from build123d import *

# Parameters (mm, degrees)
SKETCH2_R           = 27.5
BOSS_EXTRUDE1_DEPTH = 3.175
SKETCH3_R           = 1.5
SKETCH3_R_2         = 1.25
SKETCH3_W           = 3.81
SKETCH3_H           = 1.5
CUT_EXTRUDE1_DEPTH  = 3.175
SKETCH4_W           = 3.5
SKETCH4_H           = 4.54
CUT_EXTRUDE2_DEPTH  = 10
SKETCH5_W           = 19
SKETCH5_H           = 6
SKETCH5_W_2         = 12.7
SKETCH5_H_2         = 5.1
CUT_EXTRUDE3_DEPTH  = 10


with BuildPart() as part:
    # Sketch2 → Boss-Extrude1 (new body)
    with BuildSketch(Plane(origin=(0, 0, 0), x_dir=(1, 0, 0), z_dir=(0, 1, 0))):
        with Locations(Location((0, 0, 0), (0, 0, 270))):
            Circle(SKETCH2_R)
    extrude(amount=BOSS_EXTRUDE1_DEPTH)

    # Sketch3 → Cut-Extrude1 (cut)
    with BuildSketch(Plane(origin=(0, 3.175, 0), x_dir=(1, 0, 0), z_dir=(0, 1, 0))):
        with Locations((-4.7, 20.68)):
            Circle(SKETCH3_R)
        with Locations(Location((0, 15, 0), (0, 0, 270))):
            Circle(SKETCH3_R_2)
        with Locations(Location((-12.990381057, -7.5, 0), (0, 0, 270))):
            Circle(SKETCH3_R_2)
        with Locations(Location((12.990381057, -7.5, 0), (0, 0, 270))):
            Circle(SKETCH3_R_2)
        with BuildLine():
            Line((-1.90505, 20.68), (-1.90505, 22.18))
            Line((-1.90505, 22.18), (-4.7, 22.18))
            ThreePointArc((-4.7, 22.18), (-3.639339828, 21.740660172), (-3.2, 20.68))
            ThreePointArc((-3.2, 20.68), (-3.639339828, 19.619339828), (-4.7, 19.18))
            Line((-4.7, 19.18), (-1.174368952, 19.18))
            ThreePointArc((-1.174368952, 19.18), (-1.71266534, 19.845749619), (-1.90505, 20.68))
        make_face()
        with BuildLine():
            Line((1.90495, 20.68), (-1.90505, 20.68))
            ThreePointArc((-1.90505, 20.68), (-1.71266534, 19.845749619), (-1.174368952, 19.18))
            Line((-1.174368952, 19.18), (1.174268952, 19.18))
            ThreePointArc((1.174268952, 19.18), (1.71256534, 19.845749619), (1.90495, 20.68))
        make_face()
        with Locations((-5e-05, 21.43)):
            Rectangle(SKETCH3_W, SKETCH3_H)
        with BuildLine():
            Line((4.7, 22.18), (1.90495, 22.18))
            Line((1.90495, 22.18), (1.90495, 20.68))
            ThreePointArc((1.90495, 20.68), (1.71256534, 19.845749619), (1.174268952, 19.18))
            Line((1.174268952, 19.18), (4.7, 19.18))
            ThreePointArc((4.7, 19.18), (3.2, 20.68), (4.7, 22.18))
        make_face()
        with Locations((4.7, 20.68)):
            Circle(SKETCH3_R)
        with Locations((-15.55940535, -14.410319398)):
            Circle(SKETCH3_R)
        with BuildLine():
            ThreePointArc((-15.750561777, -11.079226754), (-16.027379451, -11.399040856), (-16.367944576, -11.649888379))
            Line((-16.367944576, -11.649888379), (-18.255879956, -12.739888379))
            Line((-18.255879956, -12.739888379), (-16.858443456, -15.160319398))
            ThreePointArc((-16.858443456, -15.160319398), (-16.30940535, -13.111281292), (-14.260367245, -13.660319398))
            Line((-14.260367245, -13.660319398), (-15.750561777, -11.079226754))
        make_face()
        Polygon((-18.255879956, -12.739888379), (-16.367944576, -11.649888379), (-18.272944576, -8.350331591), (-20.160879956, -9.440331591), align=None)
        with BuildLine():
            Line((-18.272944576, -8.350331591), (-16.367944576, -11.649888379))
            ThreePointArc((-16.367944576, -11.649888379), (-16.027379451, -11.399040856), (-15.750561777, -11.079226754))
            Line((-15.750561777, -11.079226754), (-17.470045712, -8.100993217))
            ThreePointArc((-17.470045712, -8.100993217), (-17.885421686, -8.180817303), (-18.272944576, -8.350331591))
        make_face()
        with BuildLine():
            Line((-20.160879956, -9.440331591), (-18.272944576, -8.350331591))
            ThreePointArc((-18.272944576, -8.350331591), (-17.885421686, -8.180817303), (-17.470045712, -8.100993217))
            Line((-17.470045712, -8.100993217), (-18.960367245, -5.519680602))
            ThreePointArc((-18.960367245, -5.519680602), (-18.810516611, -5.881452035), (-18.75940535, -6.269680602))
            ThreePointArc((-18.75940535, -6.269680602), (-19.871176783, -7.718569342), (-21.558443456, -7.019680602))
            Line((-21.558443456, -7.019680602), (-20.160879956, -9.440331591))
        make_face()
        with Locations((-20.25940535, -6.269680602)):
            Circle(SKETCH3_R)
        with BuildLine():
            ThreePointArc((17.470087928, -8.100920096), (17.888564549, -8.181681202), (18.278613112, -8.353457675))
            Line((18.278613112, -8.353457675), (20.157314831, -9.446506568))
            Line((20.157314831, -9.446506568), (21.558443456, -7.019680602))
            ThreePointArc((21.558443456, -7.019680602), (19.50940535, -7.568718708), (18.960367245, -5.519680602))
            Line((18.960367245, -5.519680602), (17.470087928, -8.100920096))
        make_face()
        Polygon((18.278613112, -8.353457675), (16.362606816, -11.646635452), (18.252304213, -12.746081749), (20.157314831, -9.446506568), align=None)
        with BuildLine():
            Line((18.252304213, -12.746081749), (16.362606816, -11.646635452))
            ThreePointArc((16.362606816, -11.646635452), (16.025165892, -11.396774761), (15.75065718, -11.079061511))
            Line((15.75065718, -11.079061511), (14.260367245, -13.660319398))
            ThreePointArc((14.260367245, -13.660319398), (15.947633918, -12.961430658), (17.05940535, -14.410319398))
            ThreePointArc((17.05940535, -14.410319398), (17.00829409, -14.798547965), (16.858443456, -15.160319398))
            Line((16.858443456, -15.160319398), (18.252304213, -12.746081749))
        make_face()
        with BuildLine():
            ThreePointArc((15.75065718, -11.079061511), (16.025165892, -11.396774761), (16.362606816, -11.646635452))
            Line((16.362606816, -11.646635452), (18.278613112, -8.353457675))
            ThreePointArc((18.278613112, -8.353457675), (17.888564549, -8.181681202), (17.470087928, -8.100920096))
            Line((17.470087928, -8.100920096), (15.75065718, -11.079061511))
        make_face()
        with Locations((15.55940535, -14.410319398)):
            Circle(SKETCH3_R)
        with Locations((20.25940535, -6.269680602)):
            Circle(SKETCH3_R)
    extrude(amount=-CUT_EXTRUDE1_DEPTH, mode=Mode.SUBTRACT)

    # Sketch4 → Cut-Extrude2 (cut)
    with BuildSketch(Plane(origin=(0, 3.175, 0), x_dir=(1, 0, 0), z_dir=(0, 1, 0))):
        Polygon((-27.104160508, -10.054216904), (-23.172405175, -7.784216904), (-24.922405175, -4.753127991), (-28.854160508, -7.023127991), align=None)
        Polygon((-22.259160508, -18.446003067), (-20.509160508, -21.47709198), (-16.577405175, -19.20709198), (-18.327405175, -16.176003067), align=None)
        with Locations((6.594873, 26.23)):
            Rectangle(SKETCH4_W, SKETCH4_H)
        with Locations((-6.595127, 26.23)):
            Rectangle(SKETCH4_W, SKETCH4_H)
        Polygon((22.259287508, -18.445783096), (18.327532175, -16.175783096), (16.577532175, -19.206872009), (20.509287508, -21.476872009), align=None)
        Polygon((27.104287508, -10.053996933), (23.172532175, -7.783996933), (24.922532175, -4.75290802), (28.854287508, -7.02290802), align=None)
    extrude(amount=-CUT_EXTRUDE2_DEPTH, mode=Mode.SUBTRACT)

    # Sketch5 → Cut-Extrude3 (cut)
    with BuildSketch(Plane(origin=(0, 3.175, 0), x_dir=(1, 0, 0), z_dir=(0, 1, 0))):
        with Locations((0, 7)):
            Rectangle(SKETCH5_W, SKETCH5_H)
        with Locations((0, -10.860319398)):
            Rectangle(SKETCH5_W_2, SKETCH5_H_2)
    extrude(amount=-CUT_EXTRUDE3_DEPTH, mode=Mode.SUBTRACT)


solid = part.part
Source: CAD feature listing. Evaluate the final solid. Frame: model axes, mm. A direction names the side the tool comes from. Give positions to 0.01 mm unless a question says otherwise; leave off trailing zeros. Order: outer loops, then holes, each group sorted by start corner. A loop starts at its lowest first (then second) coordinate and runs counter-clockwise, first axis right, second up. Notation, with made-up numbers: (58, 42) -> (91, 42) arc R24 ccw to (91, 57) -> close; hole circle Ø7 at (11, -17.75). An arc over 180 degrees is marked (long way). Use a Markdown table: item, result.
1) Ray query, line 1 along X through (y, z) = (1.35, 7.5); line 2 along Z through (x, y) = (-1, 1.9); line 3 along X through (y, z) = (2.7, 15.5). Return the intervals inside material, ascending. Write a range as [from, to].
Answer list:
| item | result |
|---|---|
| line 1 | [-23.34, -21.28], [-17.82, -14.24], [-11.74, 11.74], [14.24, 17.82], [21.28, 23.34] |
| line 2 | [-27.48, -22.18], [-19.18, -15.75], [-14.25, -10], [-4, 8.31], [13.41, 27.48] |
| line 3 | [-22.72, -16.59], [-14.53, 14.53], [16.59, 22.72] |
2) Section query C-C, the plane z = -20.68. Return the cut outline in (x, y) (3 decimals).
Answer list:
| item | result |
|---|---|
| outline | (-18.127, 0) -> (-6.2, 0) -> (-6.2, 3.175) -> (-18.127, 3.175) -> close; (6.2, 0) -> (18.127, 0) -> (18.127, 3.175) -> (6.2, 3.175) -> close |
3) Section query D-D, the plane y = 1.7. Count the separate pieces of the cut face and the enclosed holes in it, then the cut area to 3 significant figures.
Answer list:
| item | result |
|---|---|
| separate pieces | 1 |
| enclosed holes | 8 |
| area | 2,020 mm² |
4) Section query A-A, the plane x = 0. Return the cut outline in (y, z) (3 decimals), then the cut area to 3 significant figures.
Answer list:
| item | result |
|---|---|
| outline | (0, -27.5) -> (3.175, -27.5) -> (3.175, -22.18) -> (0, -22.18) -> close; (0, -19.18) -> (3.175, -19.18) -> (3.175, -16.25) -> (0, -16.25) -> close; (0, -13.75) -> (3.175, -13.75) -> (3.175, -10) -> (0, -10) -> close; (0, -4) -> (3.175, -4) -> (3.175, 8.31) -> (0, 8.31) -> close; (0, 13.41) -> (3.175, 13.41) -> (3.175, 27.5) -> (0, 27.5) -> close |
| area | 122 mm² |
5) Mould query, pull axis X, two halves, no side actions, for faces 4 (the flat face through (-25.88, 1.61, 5.306)), 5 (the flat face through (17.465, 1.61, 17.67)), 6 (the cylindrical face through (-0.3, 1.6, 27.5)), 7 (the flat face through (17.535, 1.61, 19.76)). Classes: +X half, -X half, draft (parallel to the pull), parting line (faces both ways), or undercut.
Answer list:
| item | result |
|---|---|
| face 4 | undercut |
| face 5 | undercut |
| face 6 | parting line |
| face 7 | +X half |
6) Section query B-B, the plane z = -15. Return the cut outline in (x, y) (3 decimals).
Answer list:
| item | result |
|---|---|
| outline | (-23.049, 0) -> (-1.25, 0) -> (-1.25, 3.175) -> (-23.049, 3.175) -> close; (1.25, 0) -> (23.049, 0) -> (23.049, 3.175) -> (1.25, 3.175) -> close |
7) Reachability of faces 1 (the flat face through (-4.845, 2, -25)), 2 (the flat face through (0, 2, 13.41)), 3 (the flat face through (-17.562, 1.61, 19.776)) from +Z, -Z, +X, -X, +Y, -Y: full face, straight path, thin tool, end or side. Return the list, or none.
Answer list:
| item | result |
|---|---|
| face 1 | -Z, +Y, -Y |
| face 2 | +Y, -Y |
| face 3 | -X, +Y, -Y |
8) Contact query for flat-ended pins moving along their axis: P1, Ø1, axis at y = 1, z = 10.5, coming from the +X side; P2, Ø2, axis at x = 0, z = -15, coming from the -Y side; P3, Ø1.5, axis at x = 15.5, y = 2.5, coming from the +Z side; P4, Ø0.7, axis at y = 1.5, z = -25, coming from the -X side. Output: stop coordinate, or through.
Answer list:
| item | result |
|---|---|
| P1 | x = 25.62 |
| P2 | through |
| P3 | z = 23.21 |
| P4 | x = -12.19 |
